```python
from build123d import *

# Parameters (mm, degrees)
SKETCH_1_W          = 102
SKETCH_1_H          = 67
EXTRUDE_1_DEPTH     = 3
FILLET_1_R          = 1
SKETCH_2_R          = 3
SKETCH_2_R_2        = 1.15
EXTRUDE_2_DEPTH     = 6.6
SKETCH_3_R          = 3.6
SKETCH_3_R_2        = 2.1
SKETCH_3_R_3        = 0.6
SKETCH_3_W          = 29
SKETCH_3_H          = 25
CUT_EXTRUDE_1_DEPTH = 123.215220001
CHAMFER_1_SIZE      = 1.5
CHAMFER_2_SIZE      = 0.8
SKETCH_4_R          = 1.65
CUT_EXTRUDE_2_DEPTH = 123.413888101
FILLET_2_R          = 0.6


with BuildPart() as part:
    # 草图1 → 凸台-拉伸1 (new body)
    with BuildSketch(Plane.XY):
        with Locations((51, 33.5)):
            Rectangle(SKETCH_1_W, SKETCH_1_H)
    extrude(amount=EXTRUDE_1_DEPTH)

    # 圆角1
    fillet_1_edges = [part.edges().sort_by_distance(p)[0] for p in [
        (0, 67, 1.5),
        (102, 67, 1.5),
        (102, 0, 1.5),
        (0, 0, 1.5),
    ]]
    fillet(fillet_1_edges, radius=FILLET_1_R)

    # 草图2 → 凸台-拉伸2 (add)
    # profile 1 of 4: a face of its own
    with BuildSketch(Plane.XY.offset(3)):
        with Locations(Location((15, 59, 0), (0, 0, 180))):
            Circle(SKETCH_2_R)
        with Locations((15, 59)):
            Circle(SKETCH_2_R_2, mode=Mode.SUBTRACT)
    # profile 2 of 4: a face of its own
    with BuildSketch(Plane.XY.offset(3)):
        with Locations(Location((15, 25, 0), (0, 0, 180))):
            Circle(SKETCH_2_R)
        with Locations((15, 25)):
            Circle(SKETCH_2_R_2, mode=Mode.SUBTRACT)
    # profile 3 of 4: a face of its own
    with BuildSketch(Plane.XY.offset(3)):
        with Locations(Location((69, 24.024333843, 0), (0, 0, 180))):
            Circle(SKETCH_2_R)
        with Locations((69, 24.024333843)):
            Circle(SKETCH_2_R_2, mode=Mode.SUBTRACT)
    # profile 4 of 4: a face of its own
    with BuildSketch(Plane.XY.offset(3)):
        with Locations(Location((69, 58.024333843, 0), (0, 0, 180))):
            Circle(SKETCH_2_R)
        with Locations((69, 58.024333843)):
            Circle(SKETCH_2_R_2, mode=Mode.SUBTRACT)
    extrude(amount=EXTRUDE_2_DEPTH)

    # 草图3 → 切除-拉伸1 (cut, through all)
    with BuildSketch(Plane.XY.offset(3)):
        with Locations((26.64, 34.12)):
            Circle(SKETCH_3_R)
        with Locations((18.94, 48.06)):
            Circle(SKETCH_3_R_2)
        with Locations((33.94, 48.06)):
            Circle(SKETCH_3_R_2)
        with Locations((21.7, 58.6)):
            Circle(SKETCH_3_R_3)
        with Locations((15.4, 34.13)):
            Circle(SKETCH_3_R_3)
        with BuildLine():
            Line((86.757305392, 35.144333843), (90.144398541, 35.144333843))
            ThreePointArc((90.144398541, 35.144333843), (92.000851967, 32.024333843), (90.144398541, 28.904333843))
            Line((90.144398541, 28.904333843), (86.757305392, 28.904333843))
            ThreePointArc((86.757305392, 28.904333843), (84.900851967, 32.024333843), (86.757305392, 35.144333843))
        make_face()
        with Locations((56, 41.524333843)):
            Rectangle(SKETCH_3_W, SKETCH_3_H)
        with BuildLine():
            Line((86.306453426, 55.144333843), (89.693546574, 55.144333843))
            ThreePointArc((89.693546574, 55.144333843), (91.55, 52.024333843), (89.693546574, 48.904333843))
            Line((89.693546574, 48.904333843), (86.306453426, 48.904333843))
            ThreePointArc((86.306453426, 48.904333843), (84.45, 52.024333843), (86.306453426, 55.144333843))
        make_face()
    extrude(amount=-CUT_EXTRUDE_1_DEPTH, mode=Mode.SUBTRACT)

    # 倒角1
    chamfer_1_edges = [part.edges().sort_by_distance(p)[0] for p in [
        (41.5, 41.524333843, 0),
        (56, 54.024333843, 0),
        (70.5, 41.524333843, 0),
        (56, 29.024333843, 0),
    ]]
    chamfer(chamfer_1_edges, length=CHAMFER_1_SIZE)

    # 倒角2
    chamfer_2_edges = [part.edges().sort_by_distance(p)[0] for p in [
        (84.45, 52.024333843, 0),
        (88, 55.144333843, 0),
        (91.55, 52.024333843, 0),
        (88, 48.904333843, 0),
        (84.900851967, 32.024333843, 0),
        (88.450851967, 35.144333843, 0),
        (92.000851967, 32.024333843, 0),
        (88.450851967, 28.904333843, 0),
    ]]
    chamfer(chamfer_2_edges, length=CHAMFER_2_SIZE)

    # 草图4 → 切除-拉伸2 (cut, through all)
    with BuildSketch(Plane(origin=(0, 0, 0), x_dir=(-1, 0, 0), z_dir=(0, 0, -1))):
        with Locations((-98.5, 63.5)):
            Circle(SKETCH_4_R)
        with Locations((-3.5, 63.5)):
            Circle(SKETCH_4_R)
        with Locations((-3.5, 3.5)):
            Circle(SKETCH_4_R)
        with Locations((-98.5, 3.5)):
            Circle(SKETCH_4_R)
    extrude(amount=-CUT_EXTRUDE_2_DEPTH, mode=Mode.SUBTRACT)

    # 圆角2
    fillet_2_edges = [part.edges().sort_by_distance(p)[0] for p in [
        (70.5, 54.024333843, 2.25),
        (70.5, 29.024333843, 2.25),
        (41.5, 29.024333843, 2.25),
        (41.5, 54.024333843, 2.25),
    ]]
    fillet(fillet_2_edges, radius=FILLET_2_R)


solid = part.part
```
Could you check a few things on this model? Use its own coordinates, in mm. A direction names the side the tool comes from. Coordinates: 2 decimals unless noted, no trailing zeros. Order: outer loops, then holes, each group sorted by start corner. A loop starts at its lowest first (then second) coordinate and runs counter-clockwise, first axis right, second up. Notation, with made-up numbers: M 51.5,20.5 L 96.5,20.5 A33 cw 96.5,55.5 Z; hole C 87.5,-16 d1. An arc over 180 degrees is marked long. Use a Markdown table: item, result. Add a question column.
Q1. I'm going to push flat-ended pins straight in: pin 1 (1.4 mm diameter, centred on x = 15, y = 25, fed in from +Z); pin 2 (3 mm diameter, centred on y = 56, z = 8.5, fed in from -X). Where does each tip first touch, or does it pass through?
Q2. I want a section at B-B on y = 44.5. List the corners of the cut face in (x, z) for me.
Q3. We'd pull the mould along X, two halves only. Please class faces 1 (the flat face through (102, 33, 1)), 2 (the cylindrical face through (100.15, 3.57, 1.48)), 3 (the flat face through (13.7, 59, 9.6)): pulls with the +X half, pulls with the -X half, needs draft (parallel to the pull), parting line crosses it, or undercut.
Q4. I want a section at A-A on x = 60. List the corners of the cut face in (y, z) for me, then the cut area to 3 significant figures.
Q5. Which directions (+Z, -Z, +X, -X, +Y, -Y) give clear straight access to the entire face, cutting with the end or side of a thin tool? Please do faces 4 (the cylindrical face through (71.211, 55.997, 6.254)), 5 (the conical face through (84.32, 52.08, 0.67)), 6 (the flat face through (13.7, 25, 9.6)), 7 (the flat face through (50, 0, 1)), 8 (the flat face through (88, 35.144, 2)).
Q6. I want a section at D-D on y = 63.5. List the corners of the cut face in (x, z) for me, then the cut area to 3 significant figures.
Q7. I want a section at C-C on z = 5. List the corners of the cut face in (x, y) for me, then the cut area to 3 significant figures.
Q8. If I drill on L1, parallel to Y at x = 98.5, z = 2.2; L2, parallel to Y at x = 33.94, z = 0.75; L3, parallel to X at y = 57.5, z = 7, over which ranges is the centre line in solid material (lowest first)?
Checked values:
| question | item | result |
|---|---|---|
| 1 | pin 1 | z = 3 |
| 1 | pin 2 | x = 12.4 |
| 2 | outline | M 0,0 L 40,0 L 41.5,1.5 L 41.5,3 L 0,3 Z; M 70.5,1.5 L 72,0 L 102,0 L 102,3 L 70.5,3 Z |
| 3 | face 1 | pulls with the +X half |
| 3 | face 2 | undercut |
| 3 | face 3 | needs draft |
| 4 | outline | M 0,0 L 27.52,0 L 29.02,1.5 L 29.02,3 L 0,3 Z; M 54.02,1.5 L 55.52,0 L 67,0 L 67,3 L 54.02,3 Z |
| 4 | area | 124 mm² |
| 5 | face 4 | +Z |
| 5 | face 5 | -Z |
| 5 | face 6 | +Z, +X, -X, +Y, -Y |
| 5 | face 7 | +Z, -Z, +X, -X, -Y |
| 5 | face 8 | +Z, -Z |
| 6 | outline | M 0,0 L 1.85,0 L 1.85,3 L 0,3 Z; M 5.15,0 L 96.85,0 L 96.85,3 L 5.15,3 Z; M 100.15,0 L 102,0 L 102,3 L 100.15,3 Z |
| 6 | area | 286 mm² |
| 7 | outline | C 15,25 d6; C 15,59 d6; C 69,24.02 d6; C 69,58.02 d6; hole C 15,25 d2.3; hole C 15,59 d2.3; hole C 69,24.02 d2.3; hole C 69,58.02 d2.3 |
| 7 | area | 96.5 mm² |
| 8 | L1 | 0 to 1.85, 5.15 to 61.85, 65.15 to 67 |
| 8 | L2 | 0 to 45.96, 50.16 to 67 |
| 8 | L3 | 12.4 to 17.6, 66.05 to 67.98, 70.02 to 71.95 |
